Study the drawing (mm; zero at the part's minimum x, y, z) and answer. A direction names the side the tool comes from. Round coordinates to 2 decimals unless told otherwise and drop trailing zeros. Write each loop counter-clockwise with the first axis right and the second up, starting at its lowest first coordinate (ties: lowest second). Pieces come first, ordered by that corner, then holes. Notation, with made-up numbers: (43, -16.5) - (91, -16.5) arc R20 cw to (91, -11.5) - close; hole circle Ø11 at (41, 19.25). An arc over 180 degrees is marked (long way). Return JSON: item names as keys, results as strings. Group by question number.
(1) Section D-D, the plane z = 11.5 is taken. Write down the section's boundary in (x, y), then the cut area to 3 significant figures.
(2) Section C-C, the plane z = 32 is taken. Write down the section's boundary in (x, y).
(3) Determine the mould class of the marked faces 4, 5, 6 and 7 for opening direction Z: +Z half, -Z half, draft (parallel to the pull), parting line (faces both ways), or undercut.
(4) Section A-A, the plane z = 39 is taken. Write down the section's boundary in (x, y), then the cut area to 3 significant figures.
(5) Which of the six approach directions +Z, -Z, +X, -X, +Y, -Y give full straight-line access (tool end or side, diameter ignored) to the marked faces 1, 2 and 3?
(6) Each of these flat-tipped pins is pushed along its axis until it touches: pin 1 (8 mm diameter, centred on x = 21, y = 30.5, fed in from +Z); pin 2 (7 mm diameter, centred on x = 17, z = 7, fed in from -Y); pin 3 (10 mm diameter, centred on x = 23, y = 17.5, fed in from -Z). Where does it stop, or does it pass through?
(7) Section B-B, the plane y = 14 is taken. Write down the section's boundary in (x, z).
(8) Find the intervals of material crossed by line 1 along X through (y, z) = (77.3, 39); line 2 along Z through (x, y) = (11.25, 43.15); line 3 along X through (y, z) = (49, 29.5), in increasing order. Write a range as [from, to].
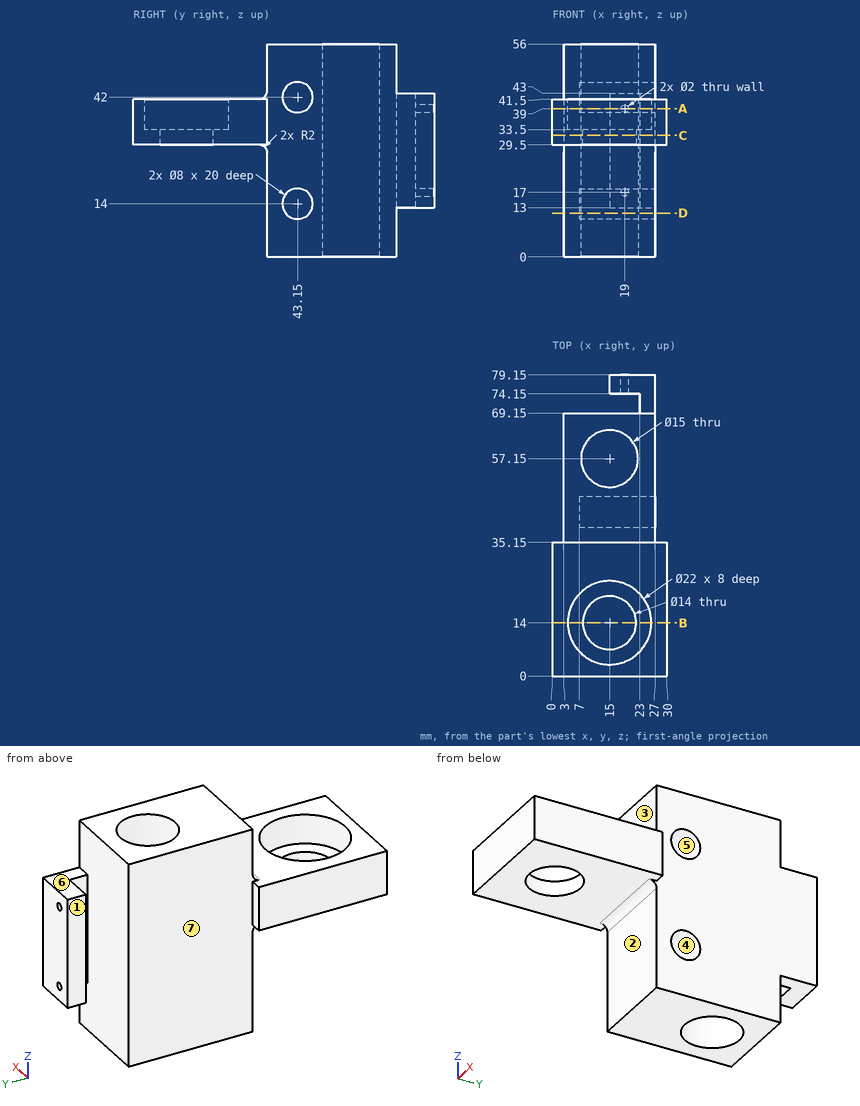
Working result:
{
 "1": {"outline": "(3, 35.15) - (27, 35.15) - (27, 40.03) - (7, 40.03) - (7, 46.27) - (27, 46.27) - (27, 69.15) - (3, 69.15) - close; hole circle Ø15 at (15, 57.15)", "area": "514 mm^2"},
 "2": {"outline": "(0, 0) - (30, 0) - (30, 35.15) - (27, 35.15) - (27, 79.15) - (15, 79.15) - (15, 74.15) - (23, 74.15) - (23, 69.15) - (3, 69.15) - (3, 35.15) - (0, 35.15) - close; hole circle Ø15 at (15, 57.15); hole circle Ø14 at (15, 14)"},
 "3": {"face 4": "undercut", "face 5": "undercut", "face 6": "+Z half", "face 7": "draft"},
 "4": {"outline": "(0, 0) - (30, 0) - (30, 35.15) - (27, 35.15) - (27, 40.5) - (7, 40.5) - (7, 45.8) - (27, 45.8) - (27, 79.15) - (20, 79.15) - (20, 74.15) - (23, 74.15) - (23, 69.15) - (3, 69.15) - (3, 35.15) - (0, 35.15) - close; (15, 74.15) - (18, 74.15) - (18, 79.15) - (15, 79.15) - close; hole circle Ø22 at (15, 14); hole circle Ø15 at (15, 57.15)", "area": "1,280 mm^2"},
 "5": {"face 1": "+Z, -Z, -X, +Y", "face 2": "-Z, +X, -X, -Y", "face 3": "+Z, +X, -X, -Y"},
 "6": {"pin 1": "stops at z = 42.02", "pin 2": "stops at y = 35.15", "pin 3": "stops at z = 29.5"},
 "7": {"outline": "(0, 29.5) - (8, 29.5) - (8, 33.5) - (4, 33.5) - (4, 41.5) - (0, 41.5) - close; (22, 29.5) - (30, 29.5) - (30, 41.5) - (26, 41.5) - (26, 33.5) - (22, 33.5) - close"},
 "8": {"line 1": "x = [15, 18], [20, 27]", "line 2": "z = [0, 10], [18, 38], [46, 56]", "line 3": "x = [3, 27]"}
}
